Build history of the part. All positions in model axes, mm. Give positions to 0.01 mm unless a question says otherwise; leave off trailing zeros. Order: outer loops, then holes, each group sorted by start corner. A loop starts at its lowest first (then second) coordinate and runs counter-clockwise, first axis right, second up. Notation, with made-up numbers: M 26.25,89.25 L 82.25,89.25 A23 cw 82.25,117.25 Z; hole C 22.5,37.5 d6. An arc over 180 degrees is marked long. One line per item, written item: value.
from build123d import *

# Parameters (mm, degrees)
F0_R     = 1.5875
F0_R_2   = 12.7
F1_DEPTH = 25.4


with BuildPart() as f1:
    # F0 (on Top) → F1 (new body)
    with BuildSketch(Plane.XY):
        with BuildLine():
            Line((38.1, -19.05), (38.1, 25.4))
            Line((38.1, 25.4), (-31.75, 25.4))
            ThreePointArc((-31.75, 25.4), (-36.240128, 23.540128), (-38.1, 19.05))
            Line((-38.1, 19.05), (-38.1, -25.4))
            Line((-38.1, -25.4), (31.75, -25.4))
            ThreePointArc((31.75, -25.4), (36.240128, -23.540128), (38.1, -19.05))
        make_face()
        with Locations((-13.470384, -13.470384)):
            Circle(F0_R, mode=Mode.SUBTRACT)
        with Locations((0, -19.05)):
            Circle(F0_R, mode=Mode.SUBTRACT)
        with Locations((-19.05, 0)):
            Circle(F0_R, mode=Mode.SUBTRACT)
        Circle(F0_R_2, mode=Mode.SUBTRACT)
        with Locations((13.470384, -13.470384)):
            Circle(F0_R, mode=Mode.SUBTRACT)
        with Locations((19.05, 0)):
            Circle(F0_R, mode=Mode.SUBTRACT)
        with Locations((-13.470384, 13.470384)):
            Circle(F0_R, mode=Mode.SUBTRACT)
        with Locations((0, 19.05)):
            Circle(F0_R, mode=Mode.SUBTRACT)
        with Locations((13.470384, 13.470384)):
            Circle(F0_R, mode=Mode.SUBTRACT)
    extrude(amount=F1_DEPTH)


solid = f1.part
1) Saw through at B-B, the plane y = -10.5. Write the cut outline in (x, z), then the cut area to 3 significant figures.
Check values:
outline: M -38.1,0 L -7.14,0 L -7.14,25.4 L -38.1,25.4 Z; M 7.14,0 L 38.1,0 L 38.1,25.4 L 7.14,25.4 Z
area: 1,570 mm^2
2) Mould opens along Y. For faces 1 (the face through (4, 25.4, 13)), 2 (the face through (-2.75, -12.4, 12.52)), 3 (the face through (8, 12, 0)), 4 (the face through (-12.004, -14.078, 12.522)) say: released by +Y, released by -Y, zero draft, split by the parting line, or undercut.
Check values:
face 1: released by +Y
face 2: undercut
face 3: zero draft
face 4: undercut
3) Pin check, flat tip, straight feed: pin 1 (3 mm diameter, centred on x = 19.05, y = 0, fed in from -Z). Stop position of the tip, or through.
Check values:
pin 1: through
4) Drill centre lines: probe 1 along Y at (x, z) = (0, 8.75); probe 2 along Y at (x, z) = (-19.05, 11); probe 3 along X at (y, z) = (14.5, 18). Where is each one in solid material? Low to high. Write a range as from..to.
Check values:
probe 1: -25.4..-20.64, -17.46..-12.7, 12.7..17.46, 20.64..25.4
probe 2: -25.4..-1.59, 1.59..25.4
probe 3: -38.1..-14.68, -12.26..12.26, 14.68..38.1
5) Saw through at C-C, the plane x = 19.05. Write the cut outline in (y, z), then the cut area to 3 significant figures.
Check values:
outline: M -25.4,0 L -1.59,0 L -1.59,25.4 L -25.4,25.4 Z; M 1.59,0 L 25.4,0 L 25.4,25.4 L 1.59,25.4 Z
area: 1,210 mm^2
6) Saw through at A-A, the plane x = 0. Write the cut outline in (y, z).
Check values:
outline: M -25.4,0 L -20.64,0 L -20.64,25.4 L -25.4,25.4 Z; M -17.46,0 L -12.7,0 L -12.7,25.4 L -17.46,25.4 Z; M 12.7,0 L 17.46,0 L 17.46,25.4 L 12.7,25.4 Z; M 20.64,0 L 25.4,0 L 25.4,25.4 L 20.64,25.4 Z
7) Saw through at D-D, the plane z = 10.75. Give the number of separate pieces and of enclosed holes in the cut face, then the cut area to 3 significant figures.
Check values:
separate pieces: 1
enclosed holes: 9
area: 3,280 mm^2
